Geometry: final body of the model. Coordinates: model frame, mm. A direction names the side the tool comes from. Give positions to 0.01 mm unless a question says otherwise; leave off trailing zeros. Order: outer loops, then holes, each group sorted by start corner. A loop starts at its lowest first (then second) coordinate and runs counter-clockwise, first axis right, second up. Notation, with made-up numbers: (53, 66.25) -> (88, 66.25) arc R21 ccw to (88, 76.25) -> close; hole circle Ø7 at (17.5, -32.75). An arc over 180 degrees is marked (long way). One line per item, written item: value. Start each with the question number.
```python
from build123d import *

# Parameters (mm, degrees)
F1_DEPTH = 7
F3_DEPTH = 1


# Not quite as in the source:
# - ends of sketch curves that miss each other by under 0.0002 mm in the source are joined


with BuildPart() as f1:
    # F0 (on Front) → F1 (new body)
    with BuildSketch(Plane.XZ):
        Polygon((-1.4500004135, 5.0060716327), (-2.9995756401, 5.0060716327), (-4.4200004135, 5.0060716327), (-4.4200004135, 7.5060716327), (-4.1678175591, 7.5060716327), (-4.4200004135, 9.0056643691), (-5.7365144081, 9.0056643691), (-5.7365144081, 2.9560173731), (-1.276, 2.9560173731), (-1.276, 2.479687877), (-4.25, 0.475687877), (0, 0.475687877), (4.25, 0.475687877), (1.276, 2.479687877), (1.276, 2.9560173731), (5.7365144081, 2.9560173731), (5.7365144081, 9.0056643691), (4.4200002068, 9.0056643691), (4.1678173524, 7.5060716327), (4.4200002068, 7.5060716327), (4.4200002068, 5.0060716327), (2.9995754333, 5.0060716327), (1.4500002068, 5.0060716327), (2.068e-07, 5.0060716327), align=None)
        Polygon((-1.4500004135, 5.8852624949), (-1.4500004135, 5.0060716327), (-4.135e-07, 5.0060716327), (1.4500002068, 5.0060716327), (1.4500002068, 5.8852624949), (2.068e-07, 5.8852624949), align=None)
    extrude(amount=F1_DEPTH)

    # F2 (on face) → F3 (cut)
    with BuildSketch(Plane(origin=(0, 0, 0), x_dir=(-1, 0, 0), z_dir=(0, 1, 0))):
        Polygon((1.276, 2.9560173731), (-1.276, 2.9560173731), (-1.276, 2.479687877), (-4.25, 0.475687877), (4.25, 0.475687877), (1.276, 2.479687877), align=None)
    extrude(amount=-F3_DEPTH, mode=Mode.SUBTRACT)


solid = f1.part
```
1. Cut plane B-B, the plane x = -2.25. Return loops of the section in (y, z), then the cut area to 3 significant figures.
2. Access query for faces 5 (the flat face through (0, -1, 1)), 6 (the flat face through (-1.45, -3.5, 5.5)), 7 (the flat face through (4.42, -3, 6)), 8 (the flat face through (-2.742, -3.958, 1.492)), 9 (the flat face through (2.784, -3.958, 1.464)). Directions: +Z, -Z, +X, -X, +Y, -Y. A direction counts if a zero-diameter tool reaches every point of the face in a straight line with its end or side. Return the directions, or none.
3. Material intervals for L1, parallel to X at y = -1, z = 5.5; L2, parallel to X at y = -4, z = 8; L3, parallel to X at y = -3, z = 6.5, sorted ascending. Write a range as [from, to].
4. Cut plane C-C, the plane y = -5.5. Return loops of the section in (x, z), then the cut area to 3 significant figures.
5. Draft query along X for faces 1 (the flat face through (5, -3, 9.006)), 2 (the flat face through (0, -3, 5.885)), 3 (the flat face through (-5.737, -3, 6)), 4 (the flat face through (-4.42, -3, 6)). Return one class per face: pulls with the +X half, pulls with the -X half, needs draft (parallel to the pull), parting line crosses it, or undercut.
6. Cut plane D-D, the plane x = -0.25. Return loops of the section in (y, z).
7. Pin query (flat end, axial travel): P1, Ø0.7, axis at x = -1, z = 2, coming from the +Y side; P2, Ø1.5, axis at x = -2.5, y = -3.5, coming from the +Z side; P3, Ø1.5, axis at x = 0, y = -5, coming from the +Z side. Return the tip coordinate at first contact, or that it passes through.
8. Cut plane A-A, the plane z = 7.25. Return loops of the section in (x, y), then the cut area to 3 significant figures.
Answers follow:
1. outline: (-7, 0.48) -> (-1, 0.48) -> (-1, 1.82) -> (-7, 1.82) -> close; (-7, 2.96) -> (0, 2.96) -> (0, 5.01) -> (-7, 5.01) -> close
1. area: 22.4 mm²
2. face 5: -Z, +X, -X, +Y
2. face 6: +Z, +Y, -Y
2. face 7: +Y, -Y
2. face 8: -X, +Y, -Y
2. face 9: +X, +Y, -Y
3. L1: x = [-5.74, -4.42], [-1.45, 1.45], [4.42, 5.74]
3. L2: x = [-5.74, -4.25], [4.25, 5.74]
3. L3: x = [-5.74, -4.42], [4.42, 5.74]
4. outline: (-5.74, 2.96) -> (-1.28, 2.96) -> (-1.28, 2.48) -> (-4.25, 0.48) -> (4.25, 0.48) -> (1.28, 2.48) -> (1.28, 2.96) -> (5.74, 2.96) -> (5.74, 9.01) -> (4.42, 9.01) -> (4.17, 7.51) -> (4.42, 7.51) -> (4.42, 5.01) -> (1.45, 5.01) -> (1.45, 5.89) -> (-1.45, 5.89) -> (-1.45, 5.01) -> (-4.42, 5.01) -> (-4.42, 7.51) -> (-4.17, 7.51) -> (-4.42, 9.01) -> (-5.74, 9.01) -> close
4. area: 49.3 mm²
5. face 1: needs draft
5. face 2: undercut
5. face 3: pulls with the -X half
5. face 4: undercut
6. outline: (-7, 0.48) -> (-1, 0.48) -> (-1, 2.96) -> (0, 2.96) -> (0, 5.89) -> (-7, 5.89) -> close
7. P1: stops at y = -1
7. P2: stops at z = 5.01
7. P3: stops at z = 5.89
8. outline: (-5.74, -7) -> (-4.42, -7) -> (-4.42, 0) -> (-5.74, 0) -> close; (4.42, -7) -> (5.74, -7) -> (5.74, 0) -> (4.42, 0) -> close
8. area: 18.4 mm²
